```python
from build123d import *

# Parameters (mm, degrees)
F1_DEPTH = 25
F3_DEPTH = 25
F4_W     = 15
F4_H     = 2.5
F5_DEPTH = 25


with BuildPart() as f1:
    # F0 (on Top) → F1 (new body)
    with BuildSketch(Plane.XY):
        Polygon((0, 15), (0, 0), (30, 0), (30, 2.5), (23.83784, 2.5), (23.83784, 12.5), (30, 12.5), (30, 15), align=None)
    extrude(amount=F1_DEPTH)

    # F2 (on face) → F3 (cut)
    with BuildSketch(Plane.XZ):
        Polygon((30, 25), (15, 25), (30, 12.5), align=None)
    extrude(amount=-F3_DEPTH, mode=Mode.SUBTRACT)

    # F4 (on face) → F5 (cut)
    with BuildSketch(Plane.XZ):
        with Locations((12.69743, 1.25)):
            Rectangle(F4_W, F4_H)
    extrude(amount=-F5_DEPTH, mode=Mode.SUBTRACT)


solid = f1.part
```
Input: part model. Units: mm. Frame: model coordinates. A direction names the side the tool comes from. Give positions to 0.01 mm unless a question says otherwise; leave off trailing zeros. Write each loop counter-clockwise with the first axis right and the second up, starting at its lowest first coordinate (ties: lowest second). Pieces come first, ordered by that corner, then holes. Notation, with made-up numbers: (-28, 1.25) - (-12, 1.25) arc R30 cw to (-12, 24.25) - close; hole circle Ø9 at (68.25, 52). An arc over 180 degrees is marked (long way). Write item = value, one per line. Start each with the question number.
1) Cut plane A-A (y = 13.25). Return loops of the section in (x, z).
2) Pin query (flat end, axial travel): pin 1 (3 mm diameter, centred on y = 7, z = 1.5, fed in from +X); pin 2 (5 mm diameter, centred on x = 9, y = 9.5, fed in from -Z); pin 3 (2 mm diameter, centred on y = 4.5, z = 0.5, fed in from -X); pin 4 (1 mm diameter, centred on x = 26.5, y = 12.5, fed in from +Z). Return the tip coordinate at first contact, or that it passes through.
3) Reachability of faces 4 (the face through (13, 7, 2.5)), 5 (the face through (3, 8, 0)), 6 (the face through (27, 2.5, 7)) from +Z, -Z, +X, -X, +Y, -Y: full face, straight path, thin tool, end or side. Return the list, or none.
4) Cut plane B-B (z = 13.5). Return loops of the section in (x, y), and give its area (3 significant figures).
5) Material intervals for L1, parallel to Y at x = 26, z = 10; L2, parallel to X at y = 6.25, z = 1; L3, parallel to Z at x = 8, y = 12.5, sorted ascending. Write a range as [from, to].
6) Cut plane C-C (x = 12.75). Return loops of the section in (y, z), and give its area (4 significant figures).
7) Cut plane D-D (z = 7.25). Return loops of the section in (x, y).
8) Draft query along X for faces 1 (the face through (21, 7, 20)), 2 (the face through (23, 8, 0)), 3 (the face through (20.197, 7, 1)). Return one class per face: pulls with the +X half, pulls with the -X half, needs draft (parallel to the pull), parting line crosses it, or undercut.
Answers follow:
q1.outline = (0, 0) - (5.2, 0) - (5.2, 2.5) - (20.2, 2.5) - (20.2, 0) - (30, 0) - (30, 12.5) - (15, 25) - (0, 25) - close
q2.pin_1 = 23.84
q2.pin_2 = 2.5
q2.pin_3 = 0
q2.pin_4 = 15.83
q3.face_4 = -Z, +Y, -Y
q3.face_5 = -Z, +X, -X, +Y, -Y
q3.face_6 = +Z, -Z, +X
q4.outline = (0, 0) - (28.8, 0) - (28.8, 2.5) - (23.84, 2.5) - (23.84, 12.5) - (28.8, 12.5) - (28.8, 15) - (0, 15) - close
q4.area = 382 mm^2
q5.L1 = [0, 2.5], [12.5, 15]
q5.L2 = [0, 5.2], [20.2, 23.84]
q5.L3 = [2.5, 25]
q6.outline = (0, 2.5) - (15, 2.5) - (15, 25) - (0, 25) - close
q6.area = 337.5 mm^2
q7.outline = (0, 0) - (30, 0) - (30, 2.5) - (23.84, 2.5) - (23.84, 12.5) - (30, 12.5) - (30, 15) - (0, 15) - close
q8.face_1 = pulls with the +X half
q8.face_2 = needs draft
q8.face_3 = undercut
